Here's how the part is built. I have some questions about the finished solid (model axes, mm). Face numbers are marked on the shaded views. A direction names the side the tool comes from. Round coordinates to 2 decimals unless told otherwise and drop trailing zeros. Write each loop counter-clockwise with the first axis right and the second up, starting at its lowest first coordinate (ties: lowest second). Pieces come first, ordered by that corner, then holes. Notation, with made-up numbers: (74.5, 29.5) - (119.5, 29.5) arc R24 cw to (119.5, 43.5) - close; hole circle Ø7 at (-1, 11.5). An arc over 180 degrees is marked (long way). One line per question, with ' | ' between items. Start each with the question number.
(1) Imagine slicing it at C-C (z = 15). Write out the boundary of the cut face in (x, y) (3 decimals), plus the area to 3 significant figures.
(2) Imagine slicing it at A-A (x = 0). Write out the boundary of the cut face in (y, z) (3 decimals), plus the area to 4 significant figures.
(3) Imagine slicing it at D-D (x = 23.5). Write out the boundary of the cut face in (y, z) (3 decimals), plus the area to 3 significant figures.
(4) For the marked faces 4, 5 and 6, which set-ups out of +Z, -Z, +X, -X, +Y, -Y let a thin tool reach every point of the face, with its end or its side?
(5) Imagine slicing it at B-B (y = 0). Write out the boundary of the cut face in (x, z) (3 decimals).
(6) If I drill on L1, parallel to X at y = 19, z = 15 (3 decimals); L2, parallel to X at y = 0, z = 22.25 (3 decimals); L3, parallel to Y at x = 0, z = 16.25 (3 decimals), over which ranges is the centre line in solid material (lowest first)?
(7) Will these pins go through, and if not, where does the flat tip stop? pin 1 (19 mm diameter, centred on x = 0.5, y = -0.5, fed in from -Z); pin 2 (5 mm diameter, centred on y = -9, z = 14, fed in from -X); pin 3 (2 mm diameter, centred on x = -21.5, z = 16.5, fed in from -Y); pin 4 (6 mm diameter, centred on x = 0, y = 0, fed in from +Z).
(8) Thinking about a two-plate mould opening in Y: for the marked faces 1, 2 and 3, which applies, pulls with the +Y half, pulls with the -Y half, needs draft (parallel to the pull), parting line crosses it, or undercut?
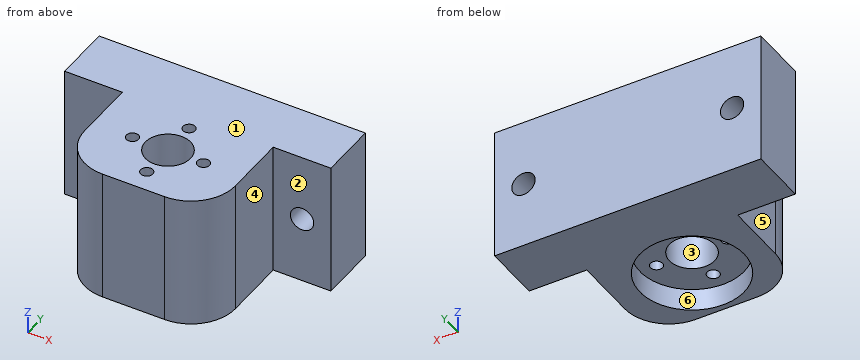
from build123d import *

# Parameters (mm, degrees)
CROQUIS1_R              = 5.1
CROQUIS1_R_2            = 1.375
SALIENTE_EXTRUIR1_DEPTH = 30
CROQUIS2_R              = 11.75
CORTAR_EXTRUIR1_DEPTH   = 5
CROQUIS3_R              = 2.625
CORTAR_EXTRUIR2_DEPTH   = 49.867806376


with BuildPart() as part:
    # Croquis1 → Saliente-Extruir1 (new body)
    with BuildSketch(Plane.XY):
        with BuildLine():
            Line((-30, 24.25), (30, 24.25))
            Line((30, 24.25), (30, 11.25))
            Line((30, 11.25), (17, 11.25))
            Line((17, 11.25), (17, -3))
            ThreePointArc((17, -3), (14.071067812, -10.071067812), (7, -13))
            Line((7, -13), (-7, -13))
            ThreePointArc((-7, -13), (-14.071067812, -10.071067812), (-17, -3))
            Line((-17, -3), (-17, 11.25))
            Line((-17, 11.25), (-30, 11.25))
            Line((-30, 11.25), (-30, 24.25))
        make_face()
        Circle(CROQUIS1_R, mode=Mode.SUBTRACT)
        with Locations((0, 8)):
            Circle(CROQUIS1_R_2, mode=Mode.SUBTRACT)
        with Locations((8, 0)):
            Circle(CROQUIS1_R_2, mode=Mode.SUBTRACT)
        with Locations((0, -8)):
            Circle(CROQUIS1_R_2, mode=Mode.SUBTRACT)
        with Locations((-8, 0)):
            Circle(CROQUIS1_R_2, mode=Mode.SUBTRACT)
    extrude(amount=SALIENTE_EXTRUIR1_DEPTH)

    # Croquis2 → Cortar-Extruir1 (cut)
    with BuildSketch(Plane(origin=(0, 0, 0), x_dir=(-1, 0, 0), z_dir=(0, 0, -1))):
        Circle(CROQUIS2_R)
    extrude(amount=-CORTAR_EXTRUIR1_DEPTH, mode=Mode.SUBTRACT)

    # Croquis3 → Cortar-Extruir2 (cut, through all)
    with BuildSketch(Plane.XZ.offset(-11.25)):
        with Locations(Location((-23.5, 15, 0), (0, 0, 270))):
            Circle(CROQUIS3_R)
        with Locations(Location((23.5, 15, 0), (0, 0, 270))):
            Circle(CROQUIS3_R)
    extrude(amount=-CORTAR_EXTRUIR2_DEPTH, mode=Mode.SUBTRACT)


solid = part.part
Check sheet entries:
1) outline: (-30, 11.25) - (-26.125, 11.25) - (-26.125, 24.25) - (-30, 24.25) - close; (-20.875, 11.25) - (-17, 11.25) - (-17, -3) arc R10 ccw to (-7, -13) - (7, -13) arc R10 ccw to (17, -3) - (17, 11.25) - (20.875, 11.25) - (20.875, 24.25) - (-20.875, 24.25) - close; (26.125, 11.25) - (30, 11.25) - (30, 24.25) - (26.125, 24.25) - close; hole circle Ø2.75 at (-8, 0); hole circle Ø10.2 at (0, 0); hole circle Ø2.75 at (0, -8); hole circle Ø2.75 at (0, 8); hole circle Ø2.75 at (8, 0) | area: 1,320 mm^2
2) outline: (-13, 0) - (-11.75, 0) - (-11.75, 5) - (-9.375, 5) - (-9.375, 30) - (-13, 30) - close; (-6.625, 5) - (-5.1, 5) - (-5.1, 30) - (-6.625, 30) - close; (5.1, 5) - (6.625, 5) - (6.625, 30) - (5.1, 30) - close; (9.375, 5) - (11.75, 5) - (11.75, 0) - (24.25, 0) - (24.25, 30) - (9.375, 30) - close | area: 607.5 mm^2
3) outline: (11.25, 0) - (24.25, 0) - (24.25, 12.375) - (11.25, 12.375) - close; (11.25, 17.625) - (24.25, 17.625) - (24.25, 30) - (11.25, 30) - close | area: 322 mm^2
4) face 4: +Z, -Z, +X, -Y | face 5: +Z, -Z, -X, -Y | face 6: -Z
5) outline: (-17, 0) - (-11.75, 0) - (-11.75, 5) - (-9.375, 5) - (-9.375, 30) - (-17, 30) - close; (-6.625, 5) - (-5.1, 5) - (-5.1, 30) - (-6.625, 30) - close; (5.1, 5) - (6.625, 5) - (6.625, 30) - (5.1, 30) - close; (9.375, 5) - (11.75, 5) - (11.75, 0) - (17, 0) - (17, 30) - (9.375, 30) - close
6) L1: -30 to -26.125, -20.875 to 20.875, 26.125 to 30 | L2: -17 to -9.375, -6.625 to -5.1, 5.1 to 6.625, 9.375 to 17 | L3: -13 to -9.375, -6.625 to -5.1, 5.1 to 6.625, 9.375 to 24.25
7) pin 1: z = 5 | pin 2: x = -16.37 | pin 3: y = 11.25 | pin 4: through
8) face 1: needs draft | face 2: pulls with the -Y half | face 3: undercut
